Autodesk Inventor part; units mm, degrees
ref_plane "YZ Plane" through (0, 0, 0) normal (1, 0, 0) x (0, 1, 0)
ref_plane "XZ Plane" through (0, 0, 0) normal (0, 1, 0) x (-1, 0, 0)
ref_plane "XY Plane" through (0, 0, 0) normal (0, 0, 1) x (1, 0, 0)
sketch "Sketch1" plane through (0, 0, 0) normal (0, 1, 0) x (-1, 0, 0)
  line L0 (25, 19.65) -> (-25, 19.65)
  line L1 (-25, 19.65) -> (-25, -19.65)
  line L2 (-25, -19.65) -> (25, -19.65)
  line L3 (25, -19.65) -> (25, 19.65)
  line L4 (25, 19.65) -> (-25, -19.65) construction
  line L5 (-25, 19.65) -> (25, -19.65) construction
  line L6 (25, 19.65) -> (-5, 19.65)
  line L7 (-5, 19.65) -> (-5, -0.35)
  line L8 (-5, -0.35) -> (25, -0.35)
  line L9 (25, -0.35) -> (25, 19.65)
  point P0 (0, 0)
  dimension "d0" = 50
  dimension "d1" = 39.3
  dimension "d2" = 30
  dimension "d3" = 20
extrude "Extrusion1" add sketch "Sketch1" along normal blind 4 contours L7 L8 L3 L2 L1 L0
properties part number "Bracket Motor Lifter_3DPrint"
Part model, mm, in its own coordinate system. A direction names the side the tool comes from. Round coordinates to 2 decimals unless told otherwise and drop trailing zeros. Loops run counter-clockwise (first coordinate to the right, second up) from the corner with the lowest first, then second, coordinate; pieces in that order, holes last. Notation, with made-up numbers: (59, 37) -> (76, 37) arc R8 cw to (76, 42) -> close; hole circle Ø5 at (-17, -23.75). An arc over 180 degrees is marked (long way). Use a Markdown table: item, result.
1) Cut at C-C, the plane z = 12.5. List the corners of the cut face in (x, y), and give its area (3 significant figures).
The answers:
| item | result |
|---|---|
| outline | (5, 0) -> (25, 0) -> (25, 4) -> (5, 4) -> close |
| area | 80.0 mm2 |
2) Drop a flat-ended pin along its axis: pin 1 Ø2 at (y, z) = (1.5, 6.5) entering from -X. Give the stop position or say it passes through.
The answers:
| item | result |
|---|---|
| pin 1 | stops at x = 5 |
3) Probe line 1 (X direction, y = 0.6, z = 7); line 2 (Z direction, x = -21.5, y = 3.55). List the from-to ranges inside material, lowest first. Write a range as [from, to].
The answers:
| item | result |
|---|---|
| line 1 | x = [5, 25] |
| line 2 | z = [-19.65, -0.35] |
4) Cut at A-A, the plane y = 3.2. List the corners of the cut face in (x, z), and give its area (4 significant figures).
The answers:
| item | result |
|---|---|
| outline | (-25, -19.65) -> (25, -19.65) -> (25, 19.65) -> (5, 19.65) -> (5, -0.35) -> (-25, -0.35) -> close |
| area | 1,365 mm2 |
5) Tool access for faces 1 (the flat face through (-10, 2, -0.35)), 2 (the flat face through (0, 2, -19.65)): list every direction of +Z, -Z, +X, -X, +Y, -Y with a clear straight run to the whole face (end or side of a thin tool).
The answers:
| item | result |
|---|---|
| face 1 | +Z, -X, +Y, -Y |
| face 2 | -Z, +X, -X, +Y, -Y |
6) Cut at B-B, the plane x = -10.5. List the corners of the cut face in (y, z), and give its area (3 significant figures).
The answers:
| item | result |
|---|---|
| outline | (0, -19.65) -> (4, -19.65) -> (4, -0.35) -> (0, -0.35) -> close |
| area | 77.2 mm2 |
